Read the model definition and answer for the solid it produces. Units are mm, in the model's axes. A direction names the side the tool comes from. Coordinates: 2 decimals unless noted, no trailing zeros. Order: outer loops, then holes, each group sorted by start corner. A loop starts at its lowest first (then second) coordinate and runs counter-clockwise, first axis right, second up. Notation, with made-up numbers: (31, -17) - (47, -17) arc R13 ccw to (47, -1) - close; hole circle Ø7 at (34.25, 40). An arc over 180 degrees is marked (long way). Write item = value, one per line.
from build123d import *

# Parameters (mm, degrees)
CLEAR_GUARD_2MM_SKETCH_R                 = 1.7
CLEAR_GUARD_2MM_DEPTH                    = 2
OPENINGS_VENT_AND_TRIM_ACCESS_SKETCH_R   = 2.45
OPENINGS_VENT_AND_TRIM_ACCESS_SKETCH_R_2 = 1.95
OPENINGS_VENT_AND_TRIM_ACCESS_DEPTH      = 2
PCB_END_STOPS_START                      = -14.5
PCB_END_STOPS_DEPTH                      = 14.5


with BuildPart() as part:
    # Clear_guard_2mm_Sketch → Clear_guard_2mm (new body)
    with BuildSketch(Plane.XY):
        with BuildLine():
            Line((-26.5, -28), (19.6, -28))
            ThreePointArc((19.6, -28), (21.014213562, -27.414213562), (21.6, -26))
            Line((21.6, -26), (21.6, 26))
            ThreePointArc((21.6, 26), (21.014213562, 27.414213562), (19.6, 28))
            Line((19.6, 28), (-26.5, 28))
            ThreePointArc((-26.5, 28), (-27.914213562, 27.414213562), (-28.5, 26))
            Line((-28.5, 26), (-28.5, -26))
            ThreePointArc((-28.5, -26), (-27.914213562, -27.414213562), (-26.5, -28))
        make_face()
        with Locations((-25.5, -23.5)):
            Circle(CLEAR_GUARD_2MM_SKETCH_R, mode=Mode.SUBTRACT)
        with Locations((18.6, -25.1)):
            Circle(CLEAR_GUARD_2MM_SKETCH_R, mode=Mode.SUBTRACT)
        with Locations((-25.5, 23.5)):
            Circle(CLEAR_GUARD_2MM_SKETCH_R, mode=Mode.SUBTRACT)
        with Locations((18.6, 25.1)):
            Circle(CLEAR_GUARD_2MM_SKETCH_R, mode=Mode.SUBTRACT)
    extrude(amount=CLEAR_GUARD_2MM_DEPTH)

    # Openings_vent_and_trim_access_Sketch → Openings_vent_and_trim_access (cut)
    with BuildSketch(Plane.XY):
        with Locations((13.2, 18)):
            Circle(OPENINGS_VENT_AND_TRIM_ACCESS_SKETCH_R)
        with Locations((-18.7, -16.58)):
            Circle(OPENINGS_VENT_AND_TRIM_ACCESS_SKETCH_R_2)
        with Locations((-18.7, -11.5)):
            Circle(OPENINGS_VENT_AND_TRIM_ACCESS_SKETCH_R_2)
        with Locations((-18.7, -6.42)):
            Circle(OPENINGS_VENT_AND_TRIM_ACCESS_SKETCH_R_2)
        with BuildLine():
            Line((-14, 6.7), (8, 6.7))
            ThreePointArc((8, 6.7), (9.3, 8), (8, 9.3))
            Line((8, 9.3), (-14, 9.3))
            ThreePointArc((-14, 9.3), (-15.3, 8), (-14, 6.7))
        make_face()
        with BuildLine():
            Line((-14, 10.7), (8, 10.7))
            ThreePointArc((8, 10.7), (9.3, 12), (8, 13.3))
            Line((8, 13.3), (-14, 13.3))
            ThreePointArc((-14, 13.3), (-15.3, 12), (-14, 10.7))
        make_face()
        with BuildLine():
            Line((-14, 14.7), (8, 14.7))
            ThreePointArc((8, 14.7), (9.3, 16), (8, 17.3))
            Line((8, 17.3), (-14, 17.3))
            ThreePointArc((-14, 17.3), (-15.3, 16), (-14, 14.7))
        make_face()
        with BuildLine():
            Line((-10, -11.3), (6, -11.3))
            ThreePointArc((6, -11.3), (7.3, -10), (6, -8.7))
            Line((6, -8.7), (-10, -8.7))
            ThreePointArc((-10, -8.7), (-11.3, -10), (-10, -11.3))
        make_face()
    extrude(amount=OPENINGS_VENT_AND_TRIM_ACCESS_DEPTH, mode=Mode.SUBTRACT)

    # PCB_end_stops_Sketch → PCB_end_stops (add)
    with BuildSketch(Plane.XY.offset(PCB_END_STOPS_START)):
        with BuildLine():
            Line((-22.7, 4.5), (-22.2, 4.5))
            ThreePointArc((-22.2, 4.5), (-21.952512627, 4.602512627), (-21.85, 4.85))
            Line((-21.85, 4.85), (-21.85, 7.95))
            ThreePointArc((-21.85, 7.95), (-21.952512627, 8.197487373), (-22.2, 8.3))
            Line((-22.2, 8.3), (-22.7, 8.3))
            ThreePointArc((-22.7, 8.3), (-22.947487373, 8.197487373), (-23.05, 7.95))
            Line((-23.05, 7.95), (-23.05, 4.85))
            ThreePointArc((-23.05, 4.85), (-22.947487373, 4.602512627), (-22.7, 4.5))
        make_face()
        with BuildLine():
            Line((-24.7, -20.6), (-24.2, -20.6))
            ThreePointArc((-24.2, -20.6), (-23.952512627, -20.497487373), (-23.85, -20.25))
            Line((-23.85, -20.25), (-23.85, -17.65))
            ThreePointArc((-23.85, -17.65), (-23.952512627, -17.402512627), (-24.2, -17.3))
            Line((-24.2, -17.3), (-24.7, -17.3))
            ThreePointArc((-24.7, -17.3), (-24.947487373, -17.402512627), (-25.05, -17.65))
            Line((-25.05, -17.65), (-25.05, -20.25))
            ThreePointArc((-25.05, -20.25), (-24.947487373, -20.497487373), (-24.7, -20.6))
        make_face()
    extrude(amount=PCB_END_STOPS_DEPTH)


solid = part.part
1) Determine the mould class of faces 1 (the face through (9.3, 8, 1)), 2 (the face through (-21.85, 6, -7)), 3 (the face through (-27.93, -27.4, 0.99)) for opening direction X: pulls with the +X half, pulls with the -X half, needs draft (parallel to the pull), parting line crosses it, or undercut.
Returned:
face_1 = undercut
face_2 = pulls with the +X half
face_3 = pulls with the -X half
2) Flat-ended cylindrical pins translate along their axes: pin 1 Ø4.5 at (x, y) = (13.2, 18) entering from -Z; pin 2 Ø0.8 at (y, z) = (-18.5, -9.5) entering from -X; pin 3 Ø1.3 at (y, z) = (-19.5, -10.5) entering from +X; pin 4 Ø12 at (x, y) = (-7.5, 6) entering from -Z. Find the tip coordinate at first contact, or state that the pin passes through.
Returned:
pin_1 = through
pin_2 = -25.05
pin_3 = -23.85
pin_4 = 0
3) For faces 4 (the face through (-3, 17.3, 1)), 5 (the face through (-24.5, -18.9, -14.5)), 6 (the face through (-25.05, -19, -7)), determine the directions among +Z, -Z, +X, -X, +Y, -Y from which every point of the face is accessible in a straight line to the end or side of a thin tool.
Returned:
face_4 = +Z, -Z
face_5 = -Z, +X, -X, +Y, -Y
face_6 = -Z, -X, +Y, -Y
4) The part is cut by section C-C (z = -5.75). Determine the outline of the cut face in (x, y), and give its area (3 significant figures).
Returned:
outline = (-25.05, -20.25) arc R0.35 ccw to (-24.7, -20.6) - (-24.2, -20.6) arc R0.35 ccw to (-23.85, -20.25) - (-23.85, -17.65) arc R0.35 ccw to (-24.2, -17.3) - (-24.7, -17.3) arc R0.35 ccw to (-25.05, -17.65) - close; (-23.05, 4.85) arc R0.35 ccw to (-22.7, 4.5) - (-22.2, 4.5) arc R0.35 ccw to (-21.85, 4.85) - (-21.85, 7.95) arc R0.35 ccw to (-22.2, 8.3) - (-22.7, 8.3) arc R0.35 ccw to (-23.05, 7.95) - close
area = 8.31 mm^2
5) Straight lines are drawn through the part: line 1 along Y through (x, z) = (-4, 0.5); line 2 along Y through (x, z) = (18.6, 1.6); line 3 along Y through (x, z) = (-18.7, 0.9). For each, find the intervals that lie inside material, in ascending order. Write a range as from..to.
Returned:
line_1 = -28..-11.3, -8.7..6.7, 9.3..10.7, 13.3..14.7, 17.3..28
line_2 = -28..-26.8, -23.4..23.4, 26.8..28
line_3 = -28..-18.53, -14.63..-13.45, -9.55..-8.37, -4.47..28
6) The part is cut by section A-A (x = -18.7). Determine the outline of the cut face in (y, z).
Returned:
outline = (-28, 0) - (-18.53, 0) - (-18.53, 2) - (-28, 2) - close; (-14.63, 0) - (-13.45, 0) - (-13.45, 2) - (-14.63, 2) - close; (-9.55, 0) - (-8.37, 0) - (-8.37, 2) - (-9.55, 2) - close; (-4.47, 0) - (28, 0) - (28, 2) - (-4.47, 2) - close
7) The part is cut by section B-B (y = 12). Determine the outline of the cut face in (x, z), and give its area (3 significant figures).
Returned:
outline = (-28.5, 0) - (-15.3, 0) - (-15.3, 2) - (-28.5, 2) - close; (9.3, 0) - (21.6, 0) - (21.6, 2) - (9.3, 2) - close
area = 51.0 mm^2
8) The part is cut by section D-D (x = -5.5). Determine the outline of the cut face in (y, z).
Returned:
outline = (-28, 0) - (-11.3, 0) - (-11.3, 2) - (-28, 2) - close; (-8.7, 0) - (6.7, 0) - (6.7, 2) - (-8.7, 2) - close; (9.3, 0) - (10.7, 0) - (10.7, 2) - (9.3, 2) - close; (13.3, 0) - (14.7, 0) - (14.7, 2) - (13.3, 2) - close; (17.3, 0) - (28, 0) - (28, 2) - (17.3, 2) - close
